Geometry: see drawing. Coordinates: mm, zero at the bounding-box minimum. Give positions to 0.01 mm unless a question says otherwise; leave off trailing zeros. Write each loop counter-clockwise with the first axis right and the second up, starting at its lowest first coordinate (ties: lowest second). Pieces come first, ordered by that corner, then holes. Notation, with made-up numbers: (3, -17.75) - (38, -17.75) arc R19 cw to (38, 12.25) - close; hole circle Ø7 at (-12, 69). An arc over 180 degrees is marked (long way). Use CSV: the item, a comma, the result in double quotes. Start each with the question number.
(1) Section D-D on x = 32.5. Output: boundary loops of the cut face in (y, z) (1 decimal).
(2) Section A-A on y = 2.6. Count the separate pieces of the cut face and the enclosed holes in it, and give its area (3 significant figures).
(3) Section C-C on x = 20. Output: boundary loops of the cut face in (y, z) (1 decimal).
(4) Line query: probe 1 along Z at (x, y) = (28, 2.1) (1 decimal); probe 2 along X at (y, z) = (2.8, 18) (1 decimal); probe 3 along Z at (x, y) = (9, 1.9) (1 decimal). Output: solid intervals per line, ascending. Write a range as [from, to].
(5) Section B-B on x = 62. Output: boundary loops of the cut face in (y, z) (1 decimal).
(6) First-contact query: pin 1 Ø1 at (x, z) = (53, 34.5) entering from +Y. Flat tip, straight axial feed; report the tip coordinate or a pass-through.
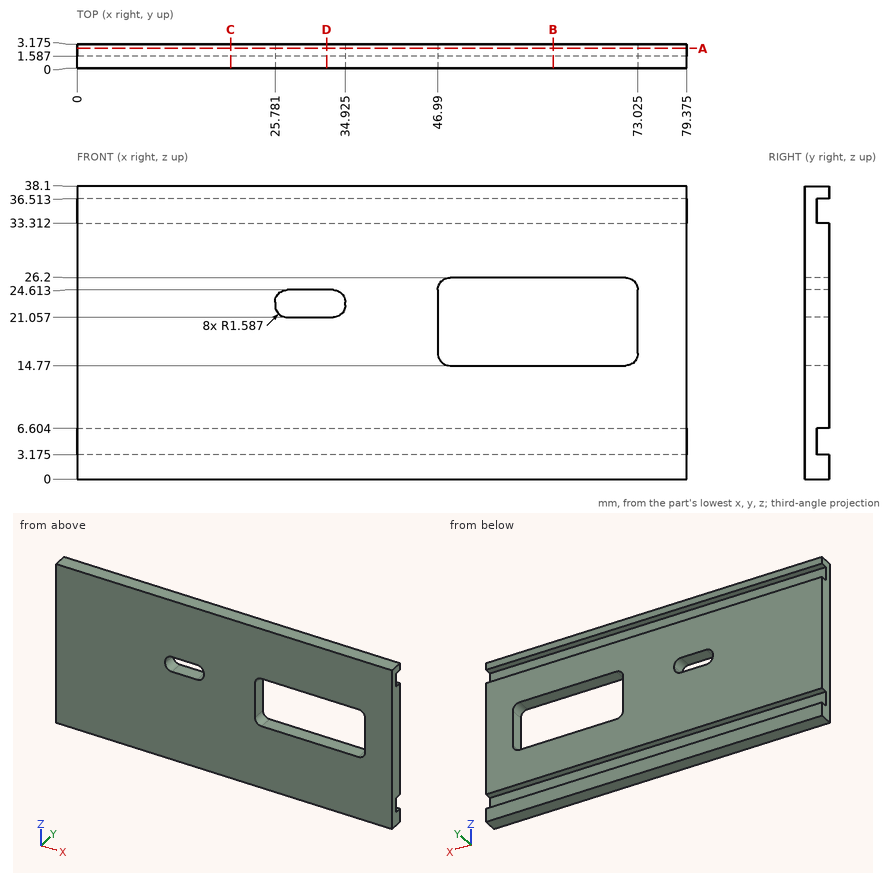
Check values:
1,outline,"(0, 0) - (3.2, 0) - (3.2, 3.2) - (1.6, 3.2) - (1.6, 6.6) - (3.2, 6.6) - (3.2, 21.1) - (0, 21.1) - close; (0, 24.6) - (3.2, 24.6) - (3.2, 33.3) - (1.6, 33.3) - (1.6, 36.5) - (3.2, 36.5) - (3.2, 38.1) - (0, 38.1) - close"
2,separate pieces,"3"
2,enclosed holes,"2"
2,area,"2,170 mm²"
3,outline,"(0, 0) - (3.2, 0) - (3.2, 3.2) - (1.6, 3.2) - (1.6, 6.6) - (3.2, 6.6) - (3.2, 33.3) - (1.6, 33.3) - (1.6, 36.5) - (3.2, 36.5) - (3.2, 38.1) - (0, 38.1) - close"
4,probe 1,"z = [0, 3.2], [6.6, 21.1], [24.6, 33.3], [36.5, 38.1]"
4,probe 2,"x = [0, 47], [73, 79.4]"
4,probe 3,"z = [0, 3.2], [6.6, 33.3], [36.5, 38.1]"
5,outline,"(0, 0) - (3.2, 0) - (3.2, 3.2) - (1.6, 3.2) - (1.6, 6.6) - (3.2, 6.6) - (3.2, 14.8) - (0, 14.8) - close; (0, 26.2) - (3.2, 26.2) - (3.2, 33.3) - (1.6, 33.3) - (1.6, 36.5) - (3.2, 36.5) - (3.2, 38.1) - (0, 38.1) - close"
6,pin 1,"stops at y = 1.59"
